from build123d import *

# Parameters (mm, degrees)
F1_DEPTH = 15
F3_DEPTH = 10
F4_R     = 2
F5_DEPTH = 25
F6_R     = 4
F7_DEPTH = 11
F8_R     = 8
F9_R     = 6
F10_R    = 3
F11_R    = 2


with BuildPart() as f1:
    # F0 (on Top) → F1 (new body)
    with BuildSketch(Plane.XY):
        Polygon((25, 0), (0, 0), (0, 25), (-10, 25), (-10, -10), (25, -10), align=None)
    extrude(amount=F1_DEPTH)

    # F2 (on face) → F3 (join)
    with BuildSketch(Plane(origin=(0, 0, 0), x_dir=(1, 0, 0), z_dir=(0, 0, -1))):
        Polygon((25, 0), (0, 0), (0, -25), (7, -25), (7, -7), (25, -7), align=None)
    extrude(amount=-F3_DEPTH)

    # F4 (on face) → F5 (cut)
    with BuildSketch(Plane.XY.offset(15)):
        with Locations((17, -5)):
            Circle(F4_R)
        with Locations((-5, 17)):
            Circle(F4_R)
    extrude(amount=-F5_DEPTH, mode=Mode.SUBTRACT)

    # F6 (on face) → F7 (cut)
    with BuildSketch(Plane.XY.offset(15)):
        with Locations((17, -5)):
            Circle(F6_R)
        with Locations((-5, 17)):
            Circle(F6_R)
    extrude(amount=-F7_DEPTH, mode=Mode.SUBTRACT)

    # F8
    f8_edges = [f1.edges().sort_by_distance(p)[0] for p in [
        (-10, -10, 7.5),
    ]]
    fillet(f8_edges, radius=F8_R)

    # F9
    f9_edges = [f1.edges().sort_by_distance(p)[0] for p in [
        (25, -10, 7.5),
        (-10, 25, 7.5),
    ]]
    fillet(f9_edges, radius=F9_R)

    # F10
    f10_edges = [f1.edges().sort_by_distance(p)[0] for p in [
        (25, 7, 5),
        (7, 7, 5),
        (7, 25, 5),
    ]]
    fillet(f10_edges, radius=F10_R)

    # F11
    f11_edges = [f1.edges().sort_by_distance(p)[0] for p in [
        (25, 0, 12.5),
        (0, 25, 12.5),
    ]]
    fillet(f11_edges, radius=F11_R)


solid = f1.part
Build history of the part. All positions in model axes, mm. A direction names the side the tool comes from. Round coordinates to 2 decimals unless told otherwise and drop trailing zeros. Write each loop counter-clockwise with the first axis right and the second up, starting at its lowest first coordinate (ties: lowest second). Pieces come first, ordered by that corner, then holes. Notation, with made-up numbers: (-27.5, -11.5) -> (23.5, -11.5) arc R33 ccw to (23.5, 19.5) -> close; hole circle Ø5 at (49, -5). An arc over 180 degrees is marked (long way). Use one line per item in the form item = value.
Q1. Band-saw the part on B-B, the plane x = 17. Write the cut outline in (y, z), then the cut area to 3 significant figures.
Conclusion:
outline = (-10, 0) -> (-7, 0) -> (-7, 4) -> (-9, 4) -> (-9, 15) -> (-10, 15) -> close; (-3, 0) -> (7, 0) -> (7, 10) -> (0, 10) -> (0, 15) -> (-1, 15) -> (-1, 4) -> (-3, 4) -> close
area = 116 mm²
Q2. Band-saw the part on D-D, the plane z = 7. Write the cut outline in (x, y).
Conclusion:
outline = (-10, -2) arc R8 ccw to (-2, -10) -> (19, -10) arc R6 ccw to (25, -4) -> (25, 4) arc R3 ccw to (22, 7) -> (10, 7) arc R3 cw to (7, 10) -> (7, 22) arc R3 ccw to (4, 25) -> (-4, 25) arc R6 ccw to (-10, 19) -> close; hole circle Ø8 at (-5, 17); hole circle Ø8 at (17, -5)
Q3. Tool access for faces 4 (the flat face through (6, 8, 10)), 5 (the flat face through (-1, 4, 15)), 6 (the flat face through (-7, 16, 4)): list every direction of +Z, -Z, +X, -X, +Y, -Y with a clear straight run to the whole face (end or side of a thin tool).
Conclusion:
face_4 = +Z, +X, +Y
face_5 = +Z, +X, -X, +Y, -Y
face_6 = +Z
Q4. Band-saw the part on C-C, the plane y = 16.5. Write the cut outline in (x, z), then the cut area to 3 significant figures.
Conclusion:
outline = (-10, 0) -> (-6.94, 0) -> (-6.94, 4) -> (-8.97, 4) -> (-8.97, 15) -> (-10, 15) -> close; (-3.06, 0) -> (7, 0) -> (7, 10) -> (0, 10) -> (0, 15) -> (-1.03, 15) -> (-1.03, 4) -> (-3.06, 4) -> close
area = 117 mm²
Q5. Two-plate mould, pull along X, no slides. Class faces 1 (the flat face through (15, -6, 4)), 2 (the flat face through (12, 0, 12)), 3 (the flat face through (0, 11, 12)): released by +X, released by -X, zero draft, split by the parting line, or undercut.
Conclusion:
face_1 = undercut
face_2 = zero draft
face_3 = released by +X
Q6. Drop flat-ended pins along their axis: P1, Ø8, axis at x = 12.5, y = 7, coming from the +Z side; P2, Ø3, axis at y = 17.5, z = 7, coming from the +X side; P3, Ø5, axis at y = -5, z = 6.5, coming from the -X side. Give the stop position or say it passes through.
Conclusion:
P1 = 10
P2 = 7
P3 = -9.98
Q7. Band-saw the part on A-A, the plane z = 2.75. Write the cut outline in (x, y), then the cut area to 3 significant figures.
Conclusion:
outline = (-10, -2) arc R8 ccw to (-2, -10) -> (19, -10) arc R6 ccw to (25, -4) -> (25, 4) arc R3 ccw to (22, 7) -> (10, 7) arc R3 cw to (7, 10) -> (7, 22) arc R3 ccw to (4, 25) -> (-4, 25) arc R6 ccw to (-10, 19) -> close; hole circle Ø4 at (-5, 17); hole circle Ø4 at (17, -5)
area = 845 mm²
Q8. Drill centre lines: L1, parallel to Y at x = 17, z = 8.25; L2, parallel to Y at x = 17, z = 13; L3, parallel to Z at x = 3, y = 14. Where is each one in solid material? Low to high.
Conclusion:
L1 = -10 to -9, -1 to 7
L2 = -10 to -9, -1 to 0
L3 = 0 to 10
